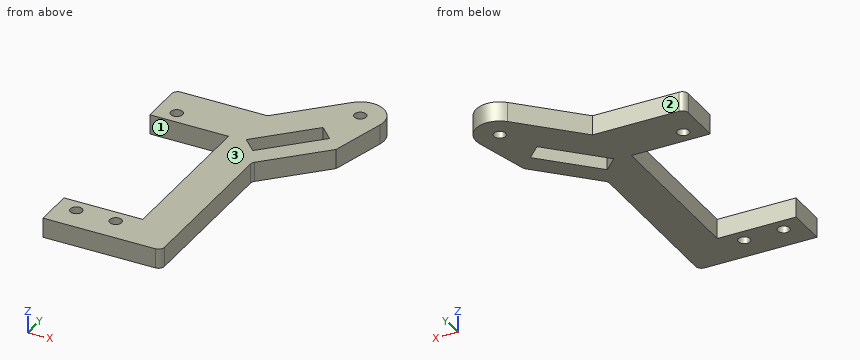
from build123d import *

# Parameters (mm, degrees)
ESQUISSE1_R        = 1.5
BOSS_EXTRU_1_DEPTH = 5
CONG_3_R           = 1.5


with BuildPart() as part:
    # Esquisse1 → Boss.-Extru.1 (new body)
    with BuildSketch(Plane.XY):
        with BuildLine():
            Line((0, 10), (0, 0))
            Line((0, 0), (30, 0))
            Line((30, 0), (30, 43.28152075))
            Line((30, 43.28152075), (43.961530357, 57.243051107))
            Line((43.961530357, 57.243051107), (47.625955008, 71.306985316))
            ThreePointArc((47.625955008, 71.306985316), (44.801829917, 78.026294211), (37.577164466, 77.06244584))
            Line((37.577164466, 77.06244584), (23.514718626, 63))
            Line((23.514718626, 63), (0, 63))
            Line((0, 63), (0, 51))
            Line((0, 51), (11, 51))
            Line((11, 51), (20, 51))
            Line((20, 51), (20, 10))
            Line((20, 10), (11, 10))
            Line((11, 10), (0, 10))
        make_face()
        with Locations((5, 54.5)):
            Circle(ESQUISSE1_R, mode=Mode.SUBTRACT)
        with Locations((15, 6.5)):
            Circle(ESQUISSE1_R, mode=Mode.SUBTRACT)
        with Locations((5, 6.5)):
            Circle(ESQUISSE1_R, mode=Mode.SUBTRACT)
        with Locations((41.819805153, 72.819805153)):
            Circle(ESQUISSE1_R, mode=Mode.SUBTRACT)
        Polygon((36.890462545, 64.314118919), (24.162540484, 51.586196858), (27.69807439, 48.050662952), (40.425996451, 60.778585013), align=None, mode=Mode.SUBTRACT)
    extrude(amount=BOSS_EXTRU_1_DEPTH)

    # Congé3
    cong_3_edges = [part.edges().sort_by_distance(p)[0] for p in [
        (30, 43.28152075, 2.5),
        (30, 0, 2.5),
        (0, 63, 2.5),
    ]]
    fillet(cong_3_edges, radius=CONG_3_R)


solid = part.part
Geometry check sheet. Reference: the model listing, model coordinates, mm. Face numbers are marked on the shaded views. A direction names the side the tool comes from. Give positions to 0.01 mm unless a question says otherwise; leave off trailing zeros. Write each loop counter-clockwise with the first axis right and the second up, starting at its lowest first coordinate (ties: lowest second). Pieces come first, ordered by that corner, then holes.
1) Thickness scan on line 1 (Y direction, x = 5, z = 2.55); line 2 (Y direction, x = 15, z = 1.6); line 3 (Y direction, x = 8.5, z = 2.95). Record the ranges inside material, lowest first.
Values follow:
line 1: y = 0 to 5, 8 to 10, 51 to 53, 56 to 63
line 2: y = 0 to 5, 8 to 10, 51 to 63
line 3: y = 0 to 10, 51 to 63
2) Cross-section at C-C (x = 15). Record the boundary of the cut face in (y, z), plus the area to 3 significant figures.
Values follow:
outline: (0, 0) - (5, 0) - (5, 5) - (0, 5) - close; (8, 0) - (10, 0) - (10, 5) - (8, 5) - close; (51, 0) - (63, 0) - (63, 5) - (51, 5) - close
area: 95.0 mm2
3) Set-up check for the marked faces 1, 2 and 3: record each of +Z, -Z, +X, -X, +Y, -Y from which the full face is reachable in a straight line by a thin tool's end or side.
Values follow:
face 1: +Z, -Z, -X
face 2: +Z, -Z, -X, +Y
face 3: +Z, +X, -X, +Y, -Y
4) Cross-section at A-A (y = 6.5). Record the boundary of the cut face in (x, z), plus the area to 3 significant figures.
Values follow:
outline: (0, 0) - (3.5, 0) - (3.5, 5) - (0, 5) - close; (6.5, 0) - (13.5, 0) - (13.5, 5) - (6.5, 5) - close; (16.5, 0) - (30, 0) - (30, 5) - (16.5, 5) - close
area: 120 mm2
5) Go/stop test with flat-tipped pins: pin 1 Ø1.5 at (y, z) = (12.5, 1.5) entering from -X; pin 2 Ø1.8 at (x, y) = (5, 54.5) entering from +Z; pin 3 Ø1 at (y, z) = (62.5, 1.5) entering from +X. Record where each tip stops, or that it passes through.
Values follow:
pin 1: stops at x = 20
pin 2: passes through
pin 3: stops at x = 45.46
6) Cross-section at B-B (x = 5). Record the boundary of the cut face in (y, z).
Values follow:
outline: (0, 0) - (5, 0) - (5, 5) - (0, 5) - close; (8, 0) - (10, 0) - (10, 5) - (8, 5) - close; (51, 0) - (53, 0) - (53, 5) - (51, 5) - close; (56, 0) - (63, 0) - (63, 5) - (56, 5) - close
7) Cross-section at D-D (z = 3.3). Record the boundary of the cut face in (x, y).
Values follow:
outline: (0, 0) - (28.5, 0) arc R1.5 ccw to (30, 1.5) - (30, 42.66) arc R1.5 cw to (30.44, 43.72) - (43.96, 57.24) - (47.63, 71.31) arc R6 ccw to (37.58, 77.06) - (23.51, 63) - (1.5, 63) arc R1.5 ccw to (0, 61.5) - (0, 51) - (20, 51) - (20, 10) - (0, 10) - close; hole circle Ø3 at (5, 6.5); hole circle Ø3 at (5, 54.5); hole circle Ø3 at (15, 6.5); hole (24.16, 51.59) - (27.7, 48.05) - (40.43, 60.78) - (36.89, 64.31) - close; hole circle Ø3 at (41.82, 72.82)
